Source: CAD feature listing. Evaluate the final solid. Frame: model axes, mm. Face numbers are marked on the shaded views. A direction names the side the tool comes from. Give positions to 0.01 mm unless a question says otherwise; leave off trailing zeros. Write each loop counter-clockwise with the first axis right and the second up, starting at its lowest first coordinate (ties: lowest second). Pieces come first, ordered by that corner, then holes. Notation, with made-up numbers: M -4.75,15.25 L 16.25,15.25 A13 ccw 16.25,26.25 Z; hole C 69,8.25 d2. An arc over 180 degrees is marked long. Use CSV: the item, a comma, the result in double quotes. Start each with the question number.
from build123d import *

# Parameters (mm, degrees)
AUFSATZ_LINEAR_AUSTRAGEN1_DEPTH = 25
SKIZZE2_W                       = 6
SKIZZE2_H                       = 1.65
AUFSATZ_LINEAR_AUSTRAGEN2_DEPTH = 8
SKIZZE3_W                       = 7.5
SKIZZE3_H                       = 0.55
SCHNITT_LINEAR_AUSTRAGEN1_DEPTH = 34
AUFSATZ_LINEAR_AUSTRAGEN3_DEPTH = 8
VERRUNDUNG1_R                   = 0.2


with BuildPart() as part:
    # Skizze1 → Aufsatz-Linear austragen1 (new body)
    with BuildSketch(Plane.XY):
        Polygon((-4.75, 0.825), (-6.7, 0.825), (-6.7, -0.825), (-4.75, -0.825), (-4.75, -3.165), (-3.75, -3.165), (-3.75, -0.825), (3.75, -0.825), (3.75, -3.165), (4.75, -3.165), (4.75, -0.825), (6.7, -0.825), (6.7, 0.825), (4.75, 0.825), (4.75, 3.165), (3.75, 3.165), (3.75, 0.825), (-3.75, 0.825), (-3.75, 3.165), (-4.75, 3.165), align=None)
    extrude(amount=AUFSATZ_LINEAR_AUSTRAGEN1_DEPTH)

    # Skizze2 → Aufsatz-Linear austragen2 (add)
    with BuildSketch(Plane(origin=(0, 0, 0), x_dir=(-1, 0, 0), z_dir=(0, 0, -1))):
        Rectangle(SKIZZE2_W, SKIZZE2_H)
    extrude(amount=AUFSATZ_LINEAR_AUSTRAGEN2_DEPTH)

    # Skizze3 → Schnitt-Linear austragen1 (cut, through all)
    with BuildSketch(Plane.XY.offset(25)):
        with Locations((0, -0.55)):
            Rectangle(SKIZZE3_W, SKIZZE3_H)
        with Locations((0, 0.55)):
            Rectangle(SKIZZE3_W, SKIZZE3_H)
    extrude(amount=-SCHNITT_LINEAR_AUSTRAGEN1_DEPTH, mode=Mode.SUBTRACT)

    # Skizze4 → Aufsatz-Linear austragen3 (add)
    with BuildSketch(Plane(origin=(0, 0, 0), x_dir=(-1, 0, 0), z_dir=(0, 0, -1))):
        Polygon((-3.75, -3.165), (-4.75, -3.165), (-4.75, -0.825), (-6.7, -0.825), (-6.7, 0.825), (-4.75, 0.825), (-4.75, 3.165), (-3.75, 3.165), (-3.75, 0.275), (-3, 0.275), (-3, -0.275), (-3.75, -0.275), align=None)
    extrude(amount=AUFSATZ_LINEAR_AUSTRAGEN3_DEPTH)

    # Verrundung1
    verrundung1_edges = [part.edges().sort_by_distance(p)[0] for p in [
        (4.25, -3.165, -8),
        (3.75, -1.72, -8),
        (3.75, 1.72, -8),
        (4.25, 3.165, -8),
        (4.75, 1.995, -8),
        (5.725, 0.825, -8),
        (6.7, 0, -8),
        (5.725, -0.825, -8),
        (4.75, -1.995, -8),
        (-4.75, -1.995, 25),
        (-4.25, -3.165, 25),
        (-5.725, 0.825, 0),
        (-4.75, 1.995, 0),
        (-4.25, 3.165, 0),
        (-3.75, -1.72, 25),
        (-4.25, -3.165, 0),
        (-4.75, -1.995, 0),
        (-5.725, -0.825, 0),
        (-6.7, 0, 0),
        (3.75, -1.72, 25),
        (4.25, -3.165, 25),
        (-6.7, 0.825, 12.5),
        (-4.75, 3.165, 12.5),
        (-3.75, 3.165, 12.5),
        (3.75, 3.165, 8.5),
        (4.75, 3.165, 8.5),
        (6.7, 0.825, 8.5),
        (6.7, -0.825, 8.5),
        (4.75, -3.165, 8.5),
        (3.75, -3.165, 8.5),
        (-3.75, -3.165, 12.5),
        (-4.75, -3.165, 12.5),
        (-6.7, -0.825, 12.5),
        (4.75, -1.995, 25),
        (5.725, -0.825, 25),
        (6.7, 0, 25),
        (5.725, 0.825, 25),
        (-6.7, 0, 25),
        (4.75, 1.995, 25),
        (4.25, 3.165, 25),
        (3.75, 1.72, 25),
        (-3.75, 1.72, 25),
        (-3, 0, -8),
        (0.375, 0.275, -8),
        (0.375, -0.275, -8),
        (-4.25, 3.165, 25),
        (-4.75, 1.995, 25),
        (-5.725, 0.825, 25),
        (0, -0.275, 25),
        (-5.725, -0.825, 25),
        (0, 0.275, 25),
    ]]
    fillet(verrundung1_edges, radius=VERRUNDUNG1_R)


solid = part.part
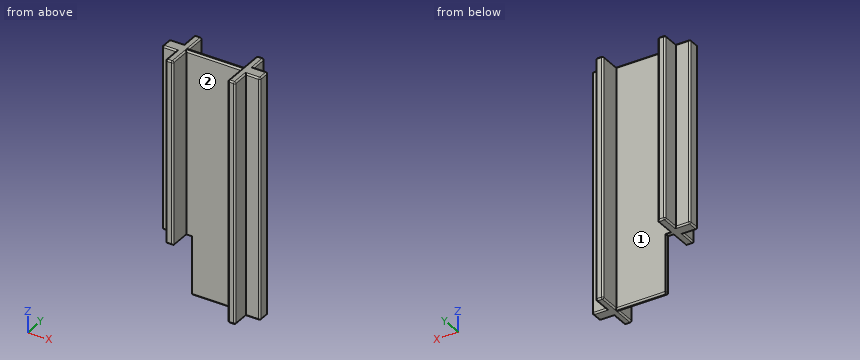
Item 1: Contact query for flat-ended pins moving along their axis: pin 1 Ø1.7 at (y, z) = (-2, 5) entering from +X; pin 2 Ø1.4 at (x, z) = (-5.5, 9.5) entering from +Y (3 decimals); pin 3 Ø1.7 at (y, z) = (2.5, 10) entering from -X. Output: stop coordinate, or through.
Item 2: Section C-C (z = -2). Return the cut outline in (x, y) (3 decimals).
Item 3: Material intervals for probe 1 along X at (y, z) = (1.5, 10); probe 2 along X at (y, z) = (0, -6.5); probe 3 along Y at (x, z) = (0.5, 20) (3 decimals), sorted ascending.
Item 4: Section B-B (x = 3). Return the cut outline in (y, z) (3 decimals), plus the area to 3 significant figures.
Item 5: Section A-A (y = 2). Return the cut outline in (x, z), plus the area to 3 significant figures.
Item 6: Set-up query: the marked faces 1 and 2. Return all of +Z, -Z, +X, -X, +Y, -Y with unobstructed straight access to the full face (end or side cutting, diameter ignored); none if empty.
Item 7: Section D-D (x = 5.5). Return the cut outline in (y, z) (3 decimals).
Output values:
1,pin 1,"stops at x = 4.75"
1,pin 2,"stops at y = 0.825"
1,pin 3,"stops at x = -4.75"
2,outline,"M -3,-0.275 L 3.75,-0.275 L 3.75,-2.965 A0.2 ccw 3.95,-3.165 L 4.55,-3.165 A0.2 ccw 4.75,-2.965 L 4.75,-0.825 L 6.5,-0.825 A0.2 ccw 6.7,-0.625 L 6.7,0.625 A0.2 ccw 6.5,0.825 L 4.75,0.825 L 4.75,2.965 A0.2 ccw 4.55,3.165 L 3.95,3.165 A0.2 ccw 3.75,2.965 L 3.75,0.275 L -3,0.275 Z"
3,probe 1,"x = -4.75 to -3.75, 3.75 to 4.75"
3,probe 2,"x = -3 to 6.7"
3,probe 3,"y = -0.275 to 0.275"
4,outline,"M -0.275,-7.8 A0.2 ccw -0.075,-8 L 0.075,-8 A0.2 ccw 0.275,-7.8 L 0.275,24.8 A0.2 ccw 0.075,25 L -0.075,25 A0.2 ccw -0.275,24.8 Z"
4,area,"18.1 mm2"
5,outline,"M -4.75,0.2 A0.2 ccw -4.55,0 L -3.75,0 L -3.75,24.8 A0.2 ccw -3.95,25 L -4.55,25 A0.2 ccw -4.75,24.8 Z; M 3.75,-7.8 A0.2 ccw 3.95,-8 L 4.55,-8 A0.2 ccw 4.75,-7.8 L 4.75,24.8 A0.2 ccw 4.55,25 L 3.95,25 A0.2 ccw 3.75,24.8 Z"
5,area,"57.9 mm2"
6,face 1,"+Z, -Z, +Y"
6,face 2,"+Z, -Z, -Y"
7,outline,"M -0.825,-7.8 A0.2 ccw -0.625,-8 L 0.625,-8 A0.2 ccw 0.825,-7.8 L 0.825,24.8 A0.2 ccw 0.625,25 L -0.625,25 A0.2 ccw -0.825,24.8 Z"
